```python
from build123d import *

# Parameters (mm, degrees)
SKETCH1_R           = 48
BOSS_EXTRUDE1_DEPTH = 12
SKETCH2_R           = 24
BOSS_EXTRUDE2_DEPTH = 10
SKETCH3_R           = 6
CUT_EXTRUDE1_DEPTH  = 34
SKETCH4_R           = 4
CUT_EXTRUDE2_DEPTH  = 10


with BuildPart() as part:
    # Sketch1 → Boss-Extrude1 (new body)
    with BuildSketch(Plane(origin=(0, 0, 0), x_dir=(1, 0, 0), z_dir=(0, 1, 0))):
        Circle(SKETCH1_R)
    extrude(amount=BOSS_EXTRUDE1_DEPTH)

    # Sketch2 → Boss-Extrude2 (add)
    with BuildSketch(Plane(origin=(0, 12, 0), x_dir=(1, 0, 0), z_dir=(0, 1, 0))):
        Circle(SKETCH2_R)
    extrude(amount=BOSS_EXTRUDE2_DEPTH)

    # Sketch3 → Cut-Extrude1 (cut)
    with BuildSketch(Plane(origin=(0, 22, 0), x_dir=(1, 0, 0), z_dir=(0, 1, 0))):
        Circle(SKETCH3_R)
    extrude(amount=-CUT_EXTRUDE1_DEPTH, mode=Mode.SUBTRACT)

    # Sketch4 → Cut-Extrude2 (cut)
    with BuildSketch(Plane.XZ):
        with Locations((0, 36)):
            Circle(SKETCH4_R)
        with Locations((31.176914536, 18)):
            Circle(SKETCH4_R)
        with Locations((31.176914536, -18)):
            Circle(SKETCH4_R)
        with Locations((0, -36)):
            Circle(SKETCH4_R)
        with Locations((-31.176914536, -18)):
            Circle(SKETCH4_R)
        with Locations((-31.176914536, 18)):
            Circle(SKETCH4_R)
    extrude(amount=-CUT_EXTRUDE2_DEPTH, mode=Mode.SUBTRACT)


solid = part.part
```
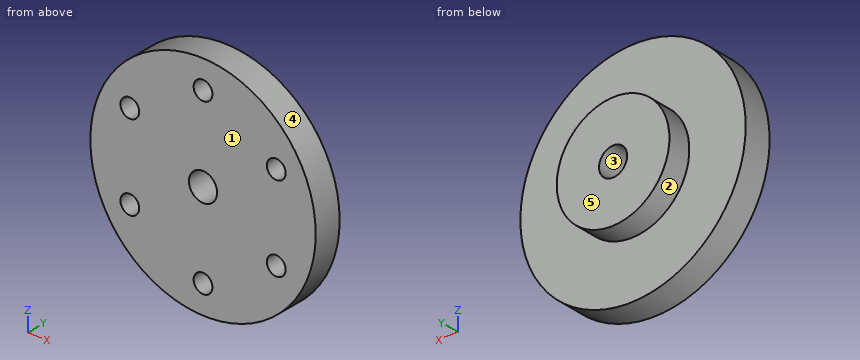
Model file for the job. Use its own axes, mm. Face numbers are marked on the shaded views. A direction names the side the tool comes from. Coordinates: 2 decimals unless noted, no trailing zeros. Order: outer loops, then holes, each group sorted by start corner. A loop starts at its lowest first (then second) coordinate and runs counter-clockwise, first axis right, second up. Notation, with made-up numbers: M -5,-27.5 L 39,-27.5 A15 cw 39,-8.5 Z; hole C 32.5,27.25 d1. An arc over 180 degrees is marked long. Answer as CSV lines item,"result".
(1) Wall check: line 1 along Z through (x, y) = (0, 2.5); line 2 along Z through (x, y) = (0, 16.5); line 3 along X through (y, z) = (1.75, -19). Give the ranges that are in metal, low to high.
Geometry says:
line 1,"z = -48 to -40, -32 to -6, 6 to 32, 40 to 48"
line 2,"z = -24 to -6, 6 to 24"
line 3,"x = -44.08 to -35.05, -27.3 to 27.3, 35.05 to 44.08"
(2) Band-saw the part on B-B, the plane x = 0. List the corners of the cut face in (y, z), then the cut area to 3 significant figures.
Geometry says:
outline,"M 0,-48 L 12,-48 L 12,-24 L 22,-24 L 22,-6 L 0,-6 L 0,-32 L 10,-32 L 10,-40 L 0,-40 Z; M 0,6 L 22,6 L 22,24 L 12,24 L 12,48 L 0,48 L 0,40 L 10,40 L 10,32 L 0,32 Z"
area,"1,210 mm2"
(3) Flat gauge pins, fed straight in: pin 1 (12 mm diameter, centred on x = 38.5, y = 3.5, fed in from +Z); pin 2 (5 mm diameter, centred on x = 0, z = -36, fed in from +Y); pin 3 (1 mm diameter, centred on y = 10.5, z = 15.5, fed in from +X). Where does each tip first touch, or does it go through?
Geometry says:
pin 1,"stops at z = 35.32"
pin 2,"stops at y = 12"
pin 3,"stops at x = 45.6"
(4) Band-saw the part on C-C, the plane z = -10. List the corners of the cut face in (x, y), then the cut area to 3 significant figures.
Geometry says:
outline,"M -46.95,0 L 46.95,0 L 46.95,12 L 21.82,12 L 21.82,22 L -21.82,22 L -21.82,12 L -46.95,12 Z"
area,"1,560 mm2"
(5) Band-saw the part on A-A, the plane z = 0. List the corners of the cut face in (x, y).
Geometry says:
outline,"M -48,0 L -6,0 L -6,22 L -24,22 L -24,12 L -48,12 Z; M 6,0 L 48,0 L 48,12 L 24,12 L 24,22 L 6,22 Z"
(6) 3-axis set-ups, long thin cutter, end or side, ignore diameter. For the marked faces 1 and 2: which of +Z, -Z, +X, -X, +Y, -Y reach the whole face in a straight line?
Geometry says:
face 1,"+Z, -Z, +X, -X, -Y"
face 2,"+Y"
(7) Pull direction Z, two halves, no side cores. Call the marked faces 3, 4 and 5: +Z half, -Z half, draft (parallel to the pull), parting line (faces both ways), or undercut.
Geometry says:
face 3,"undercut"
face 4,"parting line"
face 5,"draft"
(8) Band-saw the part on D-D, the plane z = 18. List the corners of the cut face in (x, y), then the cut area to 3 significant figures.
Geometry says:
outline,"M -44.5,0 L -35.18,0 L -35.18,10 L -27.18,10 L -27.18,0 L 27.18,0 L 27.18,10 L 35.18,10 L 35.18,0 L 44.5,0 L 44.5,12 L 15.87,12 L 15.87,22 L -15.87,22 L -15.87,12 L -44.5,12 Z"
area,"1,230 mm2"
